Build history of the part. All positions in model axes, mm. A direction names the side the tool comes from. Round coordinates to 2 decimals unless told otherwise and drop trailing zeros. Loops run counter-clockwise (first coordinate to the right, second up) from the corner with the lowest first, then second, coordinate; pieces in that order, holes last. Notation, with made-up numbers: (45, 13.25) - (78, 13.25) arc R11 cw to (78, 30.25) - close; hole circle Ø11 at (22.5, 6.25). An arc over 180 degrees is marked (long way). Use a Markdown table: item, result.
Autodesk Fusion 360 part; units mm, degrees
sketch "Sketch1" plane through (0, 0, 0) normal (0, 0, 1) x (1, 0, 0)
  line L0 (32.3278, 26.7056) -> (232.3278, 26.7056)
  line L1 (232.3278, 26.7056) -> (232.3278, 226.7056)
  line L2 (232.3278, 226.7056) -> (32.3278, 226.7056)
  line L3 (32.3278, 226.7056) -> (32.3278, 26.7056)
  dimension "d1" = 200
  dimension "d2" = 200
extrude "Extrude1" add sketch "Sketch1" along normal blind 20
sketch "Sketch2" plane through (0, 0, 20) normal (0, 0, 1) x (-1, 0, 0)
  line L0 (-32.3278, -226.7056) -> (-32.3278, -26.7056)
  line L1 (-32.3278, -26.7056) -> (-232.3278, -26.7056)
  line L2 (-232.3278, -26.7056) -> (-232.3278, -226.7056)
  line L3 (-232.3278, -226.7056) -> (-32.3278, -226.7056)
  line L4 (-232.3278, -226.7056) -> (-32.3278, -226.7056)
  line L5 (-32.3278, -226.7056) -> (-32.3278, -206.7056)
  line L6 (-32.3278, -206.7056) -> (-232.3278, -206.7056)
  line L7 (-232.3278, -206.7056) -> (-232.3278, -226.7056)
  dimension "d5" = 20
extrude "Extrude2" add sketch "Sketch2" along normal blind 100 contours L0 L2 L3 L4 L5 L6 L7
sketch "Sketch3" plane through (0, 206.7056, 0) normal (0, -1, 0) x (1, 0, 0)
  line L0 (32.3278, 20) -> (232.3278, 20)
  line L1 (232.3278, 20) -> (232.3278, 120)
  line L2 (232.3278, 120) -> (32.3278, 120)
  line L3 (32.3278, 120) -> (32.3278, 20)
  line L4 (32.3278, 120) -> (232.3278, 120)
  line L5 (232.3278, 120) -> (232.3278, 100)
  line L6 (232.3278, 100) -> (32.3278, 100)
  line L7 (32.3278, 100) -> (32.3278, 120)
  dimension "d8" = 200
  dimension "d9" = 20
extrude "Extrude3" add sketch "Sketch3" along normal blind 80 contours L1 L2 L3 L4 L5 L6 L7
sketch "Sketch4" plane through (0, 0, 20) normal (0, 0, 1) x (-1, 0, 0)
  line L0 (-232.3278, -206.7056) -> (-32.3278, -206.7056)
  line L1 (-32.3278, -206.7056) -> (-32.3278, -26.7056)
  line L2 (-32.3278, -26.7056) -> (-232.3278, -26.7056)
  line L3 (-232.3278, -26.7056) -> (-232.3278, -206.7056)
  line L4 (-232.3278, -26.7056) -> (-32.3278, -26.7056)
  line L5 (-32.3278, -26.7056) -> (-32.3278, -46.7056)
  line L6 (-32.3278, -46.7056) -> (-232.3278, -46.7056)
  line L7 (-232.3278, -46.7056) -> (-232.3278, -26.7056)
  line L8 (-232.3278, -26.7056) -> (-232.3278, -106.7056)
  line L9 (-232.3278, -106.7056) -> (-32.3278, -106.7056)
  line L10 (-32.3278, -106.7056) -> (-32.3278, -126.7056)
  line L11 (-32.3278, -126.7056) -> (-232.3278, -126.7056)
  line L12 (-232.3278, -126.7056) -> (-232.3278, -106.7056)
  dimension "d12" = 20
  dimension "d13" = 80
  dimension "d14" = 20
extrude "Extrude4" add sketch "Sketch4" along normal blind 200 contours L1 L3 L9 L10 L11 L12 | L1 L2 L3 L4 L5 L6 L7 L8
sketch "Sketch5" plane through (0, 46.7056, 0) normal (0, 1, 0) x (-1, 0, 0)
  line L0 (-232.3278, 20) -> (-32.3278, 20)
  line L1 (-32.3278, 20) -> (-32.3278, 220)
  line L2 (-32.3278, 220) -> (-232.3278, 220)
  line L3 (-232.3278, 220) -> (-232.3278, 20)
  line L4 (-232.3278, 220) -> (-32.3278, 220)
  line L5 (-32.3278, 220) -> (-32.3278, 200)
  line L6 (-32.3278, 200) -> (-232.3278, 200)
  line L7 (-232.3278, 200) -> (-232.3278, 220)
  dimension "d17" = 20
extrude "Extrude5" add sketch "Sketch5" along normal blind 60 contours L1 L2 L3 L4 L5 L6 L7
Q1. Which spindle directions (+Z, -Z, +X, -X, +Y, -Y) get a long thin tool onto all of the face, cutting with end or side? Do faces 1 (the face through (131, 126.706, 59)), 2 (the face through (232.328, 125, 87)). Say none if no direction does.
Results found:
| item | result |
|---|---|
| face 1 | +X, -X |
| face 2 | +Z, -Z, +X, +Y, -Y |
Q2. Cut at D-D, the plane z = 142. List the corners of the cut face in (x, y).
Results found:
| item | result |
|---|---|
| outline | (32.33, 26.71) - (232.33, 26.71) - (232.33, 46.71) - (32.33, 46.71) - close; (32.33, 106.71) - (232.33, 106.71) - (232.33, 126.71) - (32.33, 126.71) - close |
Q3. Cut at C-C, the plane x = 163. List the corners of the cut face in (y, z), plus the area to 3 significant figures.
Results found:
| item | result |
|---|---|
| outline | (26.71, 0) - (226.71, 0) - (226.71, 120) - (126.71, 120) - (126.71, 220) - (26.71, 220) - close; hole (46.71, 20) - (106.71, 20) - (106.71, 200) - (46.71, 200) - close; hole (126.71, 20) - (206.71, 20) - (206.71, 100) - (126.71, 100) - close |
| area | 16,800 mm2 |
Q4. Cut at B-B, the plane z = 78.5. List the corners of the cut face in (x, y), plus the area to 3 significant figures.
Results found:
| item | result |
|---|---|
| outline | (32.33, 26.71) - (232.33, 26.71) - (232.33, 46.71) - (32.33, 46.71) - close; (32.33, 106.71) - (232.33, 106.71) - (232.33, 126.71) - (32.33, 126.71) - close; (32.33, 206.71) - (232.33, 206.71) - (232.33, 226.71) - (32.33, 226.71) - close |
| area | 12,000 mm2 |
Q5. Cut at A-A, the plane y = 66. List the corners of the cut face in (x, z), plus the area to 3 significant figures.
Results found:
| item | result |
|---|---|
| outline | (32.33, 0) - (232.33, 0) - (232.33, 20) - (32.33, 20) - close; (32.33, 200) - (232.33, 200) - (232.33, 220) - (32.33, 220) - close |
| area | 8,000 mm2 |
Q6. Drop flat-ended pins along their axis: pin 1 (8 mm diameter, centred on x = 59, y = 63, fed in from -Z); pin 2 (6 mm diameter, centred on y = 151, z = 125.5, fed in from +X); pin 3 (8 mm diameter, centred on x = 145, z = 135.5, fed in from +Y). Give the stop position or say it passes through.
Results found:
| item | result |
|---|---|
| pin 1 | stops at z = 0 |
| pin 2 | passes through |
| pin 3 | stops at y = 126.71 |
Q7. Probe line 1 (Y direction, x = 164.5, z = 66); line 2 (Z direction, x = 49.5, y = 141); line 3 (Z direction, x = 170, y = 71). List the from-to ranges inside material, lowest first.
Results found:
| item | result |
|---|---|
| line 1 | y = 26.71 to 46.71, 106.71 to 126.71, 206.71 to 226.71 |
| line 2 | z = 0 to 20, 100 to 120 |
| line 3 | z = 0 to 20, 200 to 220 |
Q8. Pull direction Y, two halves, no side cores. Call faces 3 (the face through (134, 177, 120)), 4 (the face through (134, 167, 100)), 5 (the face through (131, 126.706, 169)): pulls with the +Y half, pulls with the -Y half, needs draft (parallel to the pull), parting line crosses it, or undercut.
Results found:
| item | result |
|---|---|
| face 3 | needs draft |
| face 4 | undercut |
| face 5 | pulls with the +Y half |
